```python
from build123d import *

# Parameters (mm, degrees)
F1_DEPTH = 40
F2_D     = 10
F3_R     = 5


with BuildPart() as f1:
    # F0 (on Front) → F1 (new body)
    with BuildSketch(Plane.XZ):
        with BuildLine():
            Line((-20, 55), (-20, -75))
            Line((-20, -75), (20, -75))
            Line((20, -75), (20, 55))
            ThreePointArc((20, 55), (14.1421356237, 69.1421356237), (0, 75))
            ThreePointArc((0, 75), (-14.1421356237, 69.1421356237), (-20, 55))
        make_face()
    extrude(amount=F1_DEPTH)

    # F2 (through all)
    with Locations(Plane(origin=(0, 0, 0), x_dir=(1, 0, 0), z_dir=(0, 1, 0))):
        with Locations((0, -55)):
            Hole(F2_D / 2)

    # F3
    f3_edges = [f1.edges().sort_by_distance(p)[0] for p in [
        (0, -40, 75),
        (0, 0, 75),
        (-20, 0, -10),
        (-20, -40, -10),
        (20, 0, -10),
        (20, -40, -10),
    ]]
    fillet(f3_edges, radius=F3_R)


solid = f1.part
```
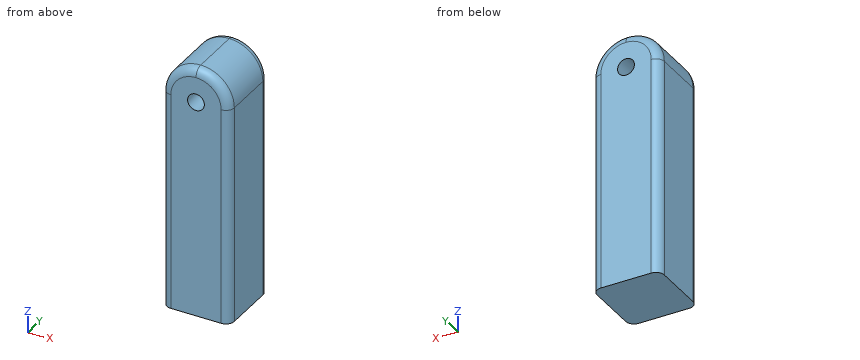
Work out the finished part from the listing and answer in its coordinate system (mm). Give positions to 0.01 mm unless a question says otherwise; leave off trailing zeros. Loops run counter-clockwise (first coordinate to the right, second up) from the corner with the lowest first, then second, coordinate; pieces in that order, holes last. Notation, with made-up numbers: M 77,50 L 99,50 A9 cw 99,64 Z; hole C 12.25,71 d3. An arc over 180 degrees is marked long. One line per item, written item: value. Start each with the question number.
1. Find the intervals of material crossed by probe 1 along Z at (x, y) = (0, -13.5); probe 2 along X at (y, z) = (-25, 55); probe 3 along Y at (x, z) = (-15.5, -51), in increasing order.
2. Find section A-A (y = -28). Give the vertices of the cut face in (x, z).
3. This flat-tipped pin is pushed along its axis until it touches: P1, Ø3, axis at x = 4.5, y = -30.5, coming from the +Z side. Where does it stop, or does it pass through?
Reported:
1. probe 1: z = -75 to 50, 60 to 75
1. probe 2: x = -20 to -5, 5 to 20
1. probe 3: y = -39.97 to -0.03
2. outline: M -20,-75 L 20,-75 L 20,55 A20 ccw -20,55 Z; hole C 0,55 d10
3. P1: stops at z = 74.77
